The model under review builds one solid part; all positions refer to its coordinate system, in mm. Face numbers are marked on the shaded views. Round coordinates to 2 decimals unless told otherwise and drop trailing zeros. Loops run counter-clockwise (first coordinate to the right, second up) from the corner with the lowest first, then second, coordinate; pieces in that order, holes last. Notation, with made-up numbers: M 3.25,72 L 47.25,72 A27 ccw 47.25,92 Z; hole C -8,89 d3. An arc over 180 degrees is marked long. One line per question, with ' | ' between items.
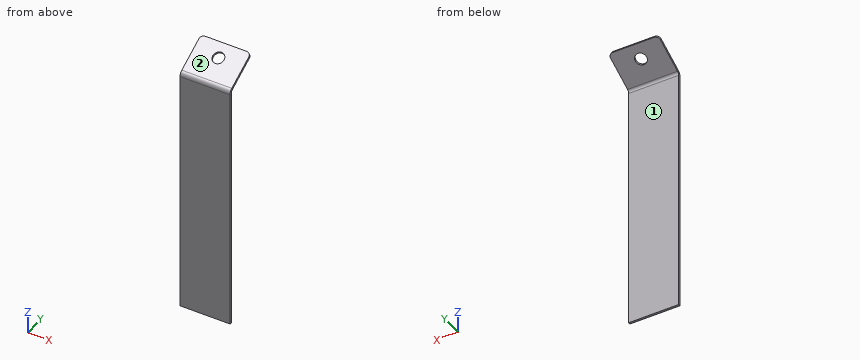
Autodesk Inventor part; units mm, degrees
ref_plane "YZ Plane" through (0, 0, 0) normal (1, 0, 0) x (0, 1, 0)
ref_plane "XZ Plane" through (0, 0, 0) normal (0, 1, 0) x (-1, 0, 0)
ref_plane "XY Plane" through (0, 0, 0) normal (0, 0, 1) x (1, 0, 0)
sketch "Sketch1" plane through (0, 0, 0) normal (0, 1, 0) x (-1, 0, 0)
  line L0 (35, 0) -> (-35, 0)
  line L1 (-35, 0) -> (-35, 343)
  line L2 (-35, 343) -> (35, 343)
  line L3 (35, 343) -> (35, 0)
  point P0 (0, 0)
  point P1 (0, 0)
  point P2 (0, 0)
  dimension "d7" = 70
  dimension "d8" = 343
extrude "Plate1" add sketch "Sketch1" along normal mid plane 3
sketch "Sketch2" plane through (35, 0, 340.4019) normal (0, -0.5, 0.8660254) x (1, 0, 0)
  line L0 (-70, 0) -> (0, 0)
  line L1 (0, 0) -> (0, 55)
  line L2 (0, 55) -> (-70, 55)
  line L3 (-70, 55) -> (-70, 0)
edge flange "Flange1" height 55 angle 60 thickness 3 bend radius 5 thickness toward (0, -0.5, 0.8660254) relief round relief width 3 relief depth 1.5 edges at (0, 1.5, 343) wall of the first edge with corners at (-35, 0, 340.4019) (35, 0, 340.4019) (35, 47.6314, 367.9019) (-35, 47.6314, 367.9019)
bend "Bend1"
corner "Corner1"
sketch "Sketch3" plane through (-35, 46.1314, 370.5) normal (0, -0.5, 0.8660254) x (1, 0, 0)
  circle A0 centre (35, -20) radius 8
  line L0 (0, 0) -> (70, 0)
  point P0 (35, -225.201)
  point P1 (35, 0)
  dimension "d19" = 20
  dimension "d20" = 16
extrude "Cut1" cut sketch "Sketch3" against normal blind 3
fillet "Corner Round1" radius 6 2 edges at (35, 46.8814, 369.201) (-35, 46.8814, 369.201)
equation "\"d21\" = Thickness"
equation "\"d6\" = Thickness"
equation "\"d9\" = BendReliefWidth"
equation "\"d10\" = BendReliefDepth"
equation "\"d11\" = MinimumRemnant"
equation "\"d12\" = TransitionRadius"
equation "\"d15\" = BendRadius"
equation "\"d16\" = CornerReliefSize"
equation "\"d17\" = GapSize"
equation "\"d18\" = JacobiRadiusSize"
equation "\"BendReliefWidth\" = Thickness"
equation "\"BendReliefDepth\" = 0.5 * Thickness"
equation "\"CornerReliefSize\" = 4 * Thickness"
equation "\"MinimumRemnant\" = 2 * Thickness"
equation "\"TransitionRadius\" = BendRadius"
equation "\"JacobiRadiusSize\" = BendRadius"
equation "\"GapSize\" = Thickness"
properties part number "MSC 202 GRID CORNER" material "Stainless Steel"
1) Insertion check: P1, Ø6, axis at x = -1.5, y = 39, coming from the +Z side; P2, Ø8, axis at x = -9, y = 6.5, coming from the +Z side; P3, Ø6, axis at x = 12, y = 34.5, coming from the -Z side. Each pin has a flat end and moves straight along its axis. Give the tip position at first contact, or say it passes through.
Output values:
P1: stops at z = 368.11 | P2: stops at z = 349.93 | P3: stops at z = 358.59
2) Add section A-A on x = -13. State the section outline as (y, z) points.
Output values:
outline: M -1.5,0 L 1.5,0 L 1.5,338.38 A5 cw 4,342.71 L 47.63,367.9 L 46.13,370.5 L 2.5,345.31 A8 ccw -1.5,338.38 Z
3) Add section D-D on y = 8.5. State the section outline as (x, z) points.
Output values:
outline: M -35,345.31 L 35,345.31 L 35,348.77 L -35,348.77 Z
4) Add section C-C on z = 174.5. State the section outline as (x, y) points, then the cut area to 3 significant figures.
Output values:
outline: M -35,-1.5 L 35,-1.5 L 35,1.5 L -35,1.5 Z | area: 210 mm²
5) Add section B-B on x = 3. State the section outline as (y, z) points.
Output values:
outline: M -1.5,0 L 1.5,0 L 1.5,338.38 A5 cw 4,342.71 L 23.89,354.19 L 22.39,356.79 L 2.5,345.31 A8 ccw -1.5,338.38 Z; M 35.23,364.21 L 36.73,361.61 L 47.63,367.9 L 46.13,370.5 Z
6) Mouldability with a two-part tool opening along Y and no side actions: class the marked faces 1 and 2 as +Y half, -Y half, draft (parallel to the pull), parting line (faces both ways), or undercut.
Output values:
face 1: +Y half | face 2: -Y half
7) For line 1 (Y direction, x = -32, z = 57); line 2 (Z direction, x = 30, y = 14); line 3 (Z direction, x = 1.5, y = 20), list the stretches that pass through material, from the lowest coordinate up.
Output values:
line 1: y = -1.5 to 1.5 | line 2: z = 348.48 to 351.95 | line 3: z = 351.95 to 355.41
